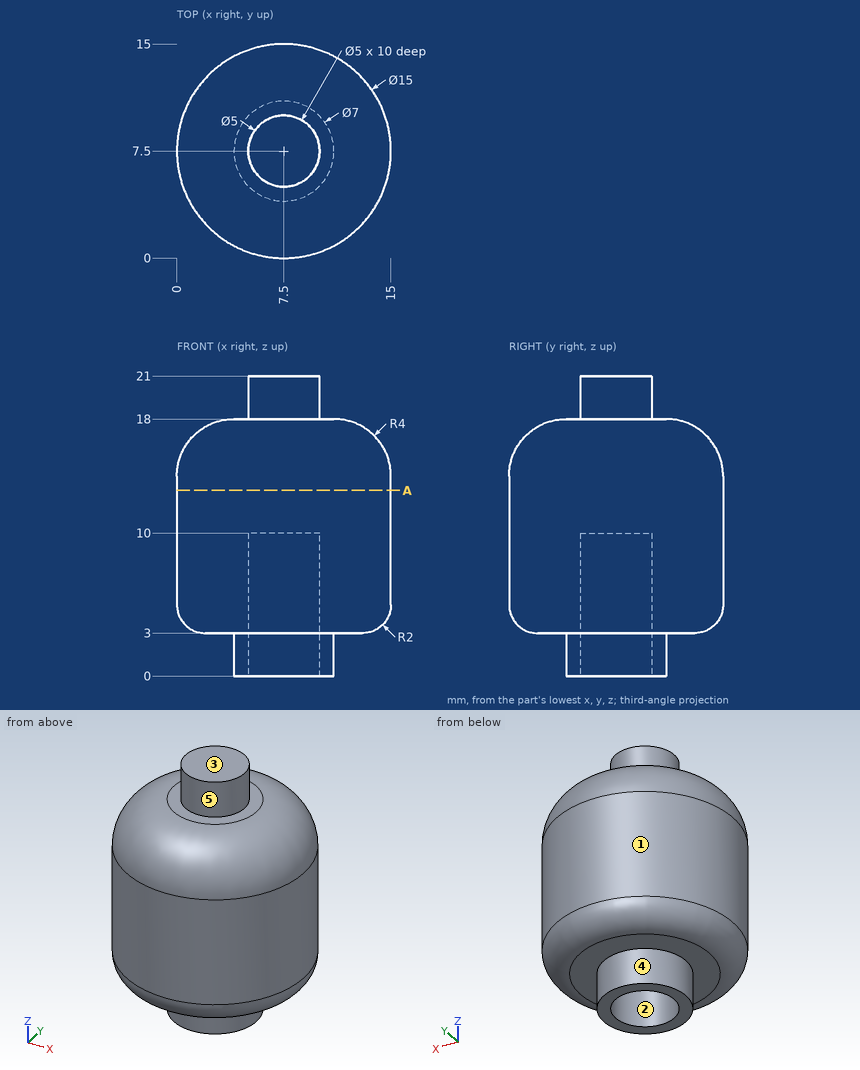
Print and shaded views of the part. All mm, measured from the part's lowest x, y and z. A direction names the side the tool comes from. Coordinates: 2 decimals unless noted, no trailing zeros. Loops run counter-clockwise (first coordinate to the right, second up) from the corner with the lowest first, then second, coordinate; pieces in that order, holes last. Notation, with made-up numbers: (2, -25.75) - (17, -25.75) arc R24 cw to (17, 7.25) - close; hole circle Ø1 at (-4.5, -29.5). An arc over 180 degrees is marked (long way). Write item = value, one per line. Start each with the question number.
Item 1: Wall check: L1, parallel to Y at x = 7.5, z = 5.5; L2, parallel to Y at x = 7.5, z = 2.5; L3, parallel to Z at x = 9.75, y = 10. Give the ranges that are in metal, low to high. Write a range as from..to.
Item 2: Mould opens along X. For the marked faces 1, 2 and 3 say: released by +X, released by -X, zero draft, split by the parting line, or undercut.
Item 3: Flat gauge pins, fed straight in: pin 1 Ø5 at (x, y) = (6, 3) entering from +Z; pin 2 Ø3 at (y, z) = (1.5, 11) entering from +X; pin 3 Ø2 at (x, y) = (10, 3.5) entering from -Z; pin 4 Ø5 at (x, z) = (2.5, 3.5) entering from +Y. Where does each tip first touch, or does it go through?
Item 4: Cut at A-A, the plane z = 13. Give the cut face in (x, y), and give its area (3 significant figures).
Item 5: 3-axis set-ups, long thin cutter, end or side, ignore diameter. For the marked faces 4 and 5: which of +Z, -Z, +X, -X, +Y, -Y reach the whole face in a straight line?
The answers:
q1.L1 = 0..5, 10..15
q1.L2 = 4..5, 10..11
q1.L3 = 0..18
q2.face_1 = split by the parting line
q2.face_2 = undercut
q2.face_3 = zero draft
q3.pin_1 = 21
q3.pin_2 = 13.5
q3.pin_3 = 3
q3.pin_4 = 14.43
q4.outline = circle Ø15 at (7.5, 7.5)
q4.area = 177 mm2
q5.face_4 = -Z
q5.face_5 = +Z
